Could you check a few things on this model? Use its own coordinates, in mm. Give positions to 0.01 mm unless a question says otherwise; leave off trailing zeros. Order: outer loops, then holes, each group sorted by start corner. A loop starts at its lowest first (then second) coordinate and runs counter-clockwise, first axis right, second up.
from build123d import *

# Parameters (mm, degrees)
SKETCH_1_R          = 6.5
EXTRUDE_1_DEPTH     = 6
FILLET_1_R          = 1
SKETCH_2_R          = 10
CUT_EXTRUDE_1_DEPTH = 5


with BuildPart() as part:
    # 草图1 → 凸台-拉伸1 (new body)
    with BuildSketch(Plane.XY):
        with BuildLine():
            Line((15, 112.5), (-15, 112.5))
            ThreePointArc((-15, 112.5), (-32.67766953, 105.17766953), (-40, 87.5))
            Line((-40, 87.5), (-40, -87.5))
            ThreePointArc((-40, -87.5), (-32.67766953, -105.17766953), (-15, -112.5))
            Line((-15, -112.5), (15, -112.5))
            ThreePointArc((15, -112.5), (32.67766953, -105.17766953), (40, -87.5))
            Line((40, -87.5), (40, 87.5))
            ThreePointArc((40, 87.5), (32.67766953, 105.17766953), (15, 112.5))
        make_face()
        with Locations((0, 57.5)):
            Circle(SKETCH_1_R, mode=Mode.SUBTRACT)
    extrude(amount=EXTRUDE_1_DEPTH)

    # 圆角1
    fillet_1_edges = [part.edges().sort_by_distance(p)[0] for p in [
        (32.67766953, -105.17766953, 6),
        (40, 0, 6),
        (32.67766953, 105.17766953, 6),
        (0, 112.5, 6),
        (-32.67766953, 105.17766953, 6),
        (-40, 0, 6),
        (-32.67766953, -105.17766953, 6),
        (0, -112.5, 6),
    ]]
    fillet(fillet_1_edges, radius=FILLET_1_R)

    # 草图2 → 切除-拉伸1 (cut)
    with BuildSketch(Plane.XY.offset(6)):
        with Locations((0, 57.5)):
            Circle(SKETCH_2_R)
    extrude(amount=-CUT_EXTRUDE_1_DEPTH, mode=Mode.SUBTRACT)


solid = part.part
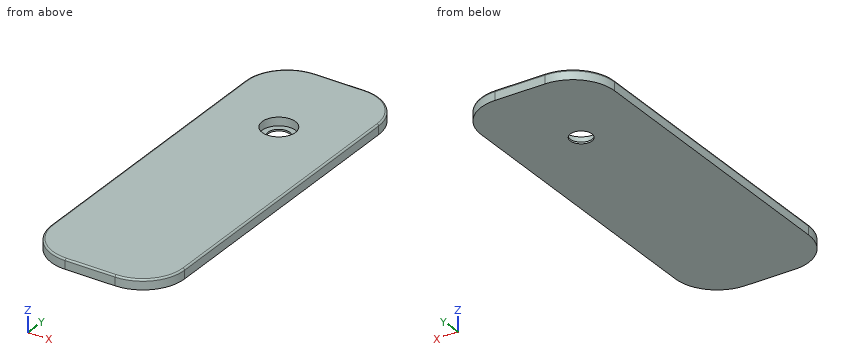
Item 1: Please list where these lines run through material, in increasing order: line 1 along Y through (x, z) = (0, 3.75); line 2 along Y through (x, z) = (0, 0.4); line 3 along X through (y, z) = (57, 1.05).
Findings:
line 1: y = -112.5 to 47.5, 67.5 to 112.5
line 2: y = -112.5 to 51, 64 to 112.5
line 3: x = -40 to -9.99, 9.99 to 40
Item 2: Imagine slicing it at B-B on y = 57.5. List the corners of the cut face in (x, z) for me.
Findings:
outline: (-40, 0) - (-6.5, 0) - (-6.5, 1) - (-10, 1) - (-10, 6) - (-39, 6) arc R1 ccw to (-40, 5) - close; (6.5, 0) - (40, 0) - (40, 5) arc R1 ccw to (39, 6) - (10, 6) - (10, 1) - (6.5, 1) - close
Item 3: For pin 1 (12 mm diameter, centred on x = 3, y = 60.5, fed in from +Z); pin 2 (16 mm diameter, centred on x = 1, y = 58, fed in from +Z); pin 3 (3 mm diameter, centred on x = 20, z = 4.5, fed in from -Y), each with a flat end and sliding along its axis, tell me the tip position at first contact or that it passes through.
Findings:
pin 1: stops at z = 6
pin 2: stops at z = 1
pin 3: stops at y = -112.25
Item 4: Imagine slicing it at C-C on z = 4.05. List the corners of the cut face in (x, y) for me.
Findings:
outline: (-40, -87.5) arc R25 ccw to (-15, -112.5) - (15, -112.5) arc R25 ccw to (40, -87.5) - (40, 87.5) arc R25 ccw to (15, 112.5) - (-15, 112.5) arc R25 ccw to (-40, 87.5) - close; hole circle Ø20 at (0, 57.5)
Item 5: Imagine slicing it at A-A on x = 0. List the corners of the cut face in (y, z) for me.
Findings:
outline: (-112.5, 0) - (51, 0) - (51, 1) - (47.5, 1) - (47.5, 6) - (-111.5, 6) arc R1 ccw to (-112.5, 5) - close; (64, 0) - (112.5, 0) - (112.5, 5) arc R1 ccw to (111.5, 6) - (67.5, 6) - (67.5, 1) - (64, 1) - close
